```python
from build123d import *

# Parameters (mm, degrees)
BOSS_EXTRUDE1_DEPTH = 4.7625
SKETCH2_R           = 16.764
SKETCH2_R_2         = 2.2225
SKETCH2_W           = 17.78
SKETCH2_H           = 6.35
SKETCH2_W_2         = 39.37
SKETCH2_H_2         = 7.112
CUT_EXTRUDE1_DEPTH  = 309.122058256
SKETCH3_W           = 63.5
SKETCH3_H           = 4.7625
BOSS_EXTRUDE2_DEPTH = 4.7625


with BuildPart() as part:
    # Sketch1 → Boss-Extrude1 (new body)
    with BuildSketch(Plane(origin=(0, 0, 0), x_dir=(1, 0, 0), z_dir=(0, 1, 0))):
        Polygon((63.5, 0), (-63.5, 0), (-20.325994648, 301.470183232), (20.325994648, 301.470183232), align=None)
    extrude(amount=BOSS_EXTRUDE1_DEPTH)

    # Sketch2 → Cut-Extrude1 (cut, through all)
    with BuildSketch(Plane(origin=(0, 4.7625, 0), x_dir=(1, 0, 0), z_dir=(0, 1, 0))):
        with Locations(Location((0, 38.862, 0), (0, 0, 270))):
            Circle(SKETCH2_R)
        with Locations(Location((-11.43, 78.359, 0), (0, 0, 270))):
            Circle(SKETCH2_R_2)
        with Locations(Location((11.43, 78.359, 0), (0, 0, 270))):
            Circle(SKETCH2_R_2)
        with Locations((0, 298.295183232)):
            Rectangle(SKETCH2_W, SKETCH2_H)
        with Locations((0, 195.58)):
            Rectangle(SKETCH2_W_2, SKETCH2_H_2)
    extrude(amount=-CUT_EXTRUDE1_DEPTH, mode=Mode.SUBTRACT)

    # Sketch3 → Boss-Extrude2 (add)
    with BuildSketch(Plane.XY):
        with Locations((0, 2.38125)):
            Rectangle(SKETCH3_W, SKETCH3_H)
    extrude(amount=BOSS_EXTRUDE2_DEPTH)


solid = part.part
```
The model under review builds one solid part; all positions refer to its coordinate system, in mm. Coordinates: 2 decimals unless noted, no trailing zeros. Write each loop counter-clockwise with the first axis right and the second up, starting at its lowest first coordinate (ties: lowest second). Pieces come first, ordered by that corner, then holes. Notation, with made-up numbers: (75.5, 30) - (108.5, 30) arc R4 cw to (108.5, 35) - close; hole circle Ø8 at (-21, 71). An arc over 180 degrees is marked (long way). Write item = value, one per line.
(1) Consider section D-D, the plane x = -41. Give the boundary of the cut face in (y, z).
Result sheet:
outline = (0, -157.11) - (4.76, -157.11) - (4.76, 0) - (0, 0) - close
(2) Consider section A-A, the plane y = 1.9. State how many separate pieces and enclosed holes the cut face has, then the cut area to 3 significant figures.
Result sheet:
separate_pieces = 1
enclosed_holes = 4
area = 24,300 mm^2
(3) Mouldability with a two-part tool opening along X and no side actions: class faces 1 (the face through (1, 0, -116)), 2 (the face through (-42.215, 2.348, -148.625)), 3 (the face through (-10.201, 2.415, -52.165)) as pulls with the +X half, pulls with the -X half, needs draft (parallel to the pull), parting line crosses it, or undercut.
Result sheet:
face_1 = needs draft
face_2 = pulls with the -X half
face_3 = undercut
(4) For P1, Ø1.4, axis at y = 1.5, z = 3.5, coming from the +X side; P2, Ø1, axis at x = -2.5, y = 0.5, coming from the -Z side; P3, Ø1.4, axis at y = 2, z = -196.5, coming from the +X side, all flat-tipped, find the tip position at first contact; note any pin that passes through.
Result sheet:
P1 = 31.75
P2 = -295.12
P3 = 35.46
(5) Consider section C-C, the plane z = -244. Give the boundary of the cut face in (x, y).
Result sheet:
outline = (-28.56, 0) - (28.56, 0) - (28.56, 4.76) - (-28.56, 4.76) - close
(6) For line 1 (Z direction, x = -1, y = 1.5); line 2 (Z direction, x = -2.5, y = 2.4); line 3 (Z direction, x = 12, y = 3.75), list the stretches that pass through material, from the lowest coordinate up. Write a range as [from, to].
Result sheet:
line_1 = [-295.12, -199.14], [-192.02, -55.6], [-22.13, 4.76]
line_2 = [-295.12, -199.14], [-192.02, -55.44], [-22.29, 4.76]
line_3 = [-301.47, -199.14], [-192.02, -80.51], [-76.21, -50.57], [-27.16, 4.76]
(7) Consider section B-B, the plane x = 5. Give the boundary of the cut face in (y, z), then the cut area to 3 significant figures.
Result sheet:
outline = (0, -295.12) - (4.76, -295.12) - (4.76, -199.14) - (0, -199.14) - close; (0, -192.02) - (4.76, -192.02) - (4.76, -54.86) - (0, -54.86) - close; (0, -22.86) - (4.76, -22.86) - (4.76, 4.76) - (0, 4.76) - close
area = 1,240 mm^2
